from build123d import *

# Parameters (mm, degrees)
BOSS_EXTRUDE1_DEPTH            = 3
F_6_1_6_1_DIAMETER_HOLE1_D     = 6.1
F_6_1_6_1_DIAMETER_HOLE1_DEPTH = 10
F_6_1_6_1_DIAMETER_HOLE1_TIP   = 1.832624888


with BuildPart() as part:
    # Sketch1 → Boss-Extrude1 (new body)
    with BuildSketch(Plane.XY):
        with BuildLine():
            Line((0, 25), (0, 14.95))
            Line((0, 14.95), (-3, 14.95))
            Line((-3, 14.95), (-3, 5))
            Line((-3, 5), (0, 5))
            Line((0, 5), (0, -5))
            Line((0, -5), (-3, -5))
            Line((-3, -5), (-3, -14.95))
            Line((-3, -14.95), (0, -14.95))
            Line((0, -14.95), (0, -25))
            ThreePointArc((0, -25), (9.091095991, -23.288451509), (16.937403852, -18.388157895))
            ThreePointArc((16.937403852, -18.388157895), (21.017483939, -15.840005215), (25.744853855, -14.95))
            Line((25.744853855, -14.95), (45, -14.95))
            ThreePointArc((45, -14.95), (54.192388155, -11.142388155), (58, -1.95))
            Line((58, -1.95), (58, 1.95))
            ThreePointArc((58, 1.95), (54.192388155, 11.142388155), (45, 14.95))
            Line((45, 14.95), (25.744853855, 14.95))
            ThreePointArc((25.744853855, 14.95), (21.017483939, 15.840005215), (16.937403852, 18.388157895))
            ThreePointArc((16.937403852, 18.388157895), (9.091095991, 23.288451509), (0, 25))
        make_face()
    extrude(amount=BOSS_EXTRUDE1_DEPTH)

    # Ø6.1 (6.1) Diameter Hole1
    with Locations(Plane.XY.offset(3)):
        with Locations((10.1, 0), (45, 0)):
            Hole(F_6_1_6_1_DIAMETER_HOLE1_D / 2, depth=F_6_1_6_1_DIAMETER_HOLE1_DEPTH)
            with Locations((0, 0, -(F_6_1_6_1_DIAMETER_HOLE1_DEPTH + F_6_1_6_1_DIAMETER_HOLE1_TIP / 2))):  # 118° drill point
                Cone(0, F_6_1_6_1_DIAMETER_HOLE1_D / 2, F_6_1_6_1_DIAMETER_HOLE1_TIP, mode=Mode.SUBTRACT)


solid = part.part
Input: part model. Units: mm. Frame: model coordinates. A direction names the side the tool comes from. Coordinates: 2 decimals unless noted, no trailing zeros. Order: outer loops, then holes, each group sorted by start corner. A loop starts at its lowest first (then second) coordinate and runs counter-clockwise, first axis right, second up. Notation, with made-up numbers: M 39,57.25 L 74,57.25 A21 cw 74,68.25 Z; hole C 74,48 d7. An arc over 180 degrees is marked long. One line per question, with ' | ' between items.
Item 1: Section B-B (z = 1). Output: boundary loops of the cut face in (x, y), then the cut area to 3 significant figures.
Geometry results:
outline: M -3,-14.95 L 0,-14.95 L 0,-25 A25 ccw 16.94,-18.39 A13 cw 25.74,-14.95 L 45,-14.95 A13 ccw 58,-1.95 L 58,1.95 A13 ccw 45,14.95 L 25.74,14.95 A13 cw 16.94,18.39 A25 ccw 0,25 L 0,14.95 L -3,14.95 L -3,5 L 0,5 L 0,-5 L -3,-5 Z; hole C 10.1,0 d6.1; hole C 45,0 d6.1 | area: 1,950 mm^2
Item 2: Reachability of faces 1 (the flat face through (0, 20, 1)), 2 (the flat face through (-2, 5, 1)), 3 (the flat face through (-2, -14.95, 1)) from +Z, -Z, +X, -X, +Y, -Y: full face, straight path, thin tool, end or side. Return the list, or none.
Geometry results:
face 1: +Z, -Z, -X, +Y | face 2: +Z, -Z, -X | face 3: +Z, -Z, -X, -Y
Item 3: Pin query (flat end, axial travel): pin 1 (1.5 mm diameter, centred on y = -1.5, z = 2, fed in from -X); pin 2 (1.5 mm diameter, centred on x = 10.5, z = 1, fed in from +Y); pin 3 (0.9 mm diameter, centred on x = -1, z = 1, fed in from -Y). Return the tip coordinate at first contact, or that it passes through.
Geometry results:
pin 1: stops at x = 0 | pin 2: stops at y = 23.02 | pin 3: stops at y = -14.95
Item 4: Ray query, line 1 along X through (y, z) = (-0.5, 1.45); line 2 along Y through (x, z) = (45, 1.35); line 3 along Y through (x, z) = (26.5, 1.25). Return the intervals inside material, ascending.
Geometry results:
line 1: x = 0 to 7.09, 13.11 to 41.99, 48.01 to 58 | line 2: y = -14.95 to -3.05, 3.05 to 14.95 | line 3: y = -14.95 to 14.95
Item 5: Section C-C (x = 12). Output: boundary loops of the cut face in (y, z).
Geometry results:
outline: M -21.93,0 L -2.39,0 L -2.39,3 L -21.93,3 Z; M 2.39,0 L 21.93,0 L 21.93,3 L 2.39,3 Z
Item 6: Draft query along X for faces 4 (the cylindrical face through (20.954, -15.865, 1.479)), 5 (the cylindrical face through (7.19, 0.92, 1.48)), 6 (the flat face through (36, 14.95, 1)). Return one class per face: released by +X, released by -X, zero draft, split by the parting line, or undercut.
Geometry results:
face 4: released by +X | face 5: undercut | face 6: zero draft
Item 7: Section D-D (y = 13). Output: boundary loops of the cut face in (x, z), then the cut area to 3 significant figures.
Geometry results:
outline: M -3,0 L 51.85,0 L 51.85,3 L -3,3 Z | area: 165 mm^2
Item 8: Section A-A (y = 0). Output: boundary loops of the cut face in (x, z).
Geometry results:
outline: M 0,0 L 7.05,0 L 7.05,3 L 0,3 Z; M 13.15,0 L 41.95,0 L 41.95,3 L 13.15,3 Z; M 48.05,0 L 58,0 L 58,3 L 48.05,3 Z
